from build123d import *

# Parameters (mm, degrees)
SKETCH1_W           = 38
SKETCH1_H           = 38
SKETCH1_R           = 1
BOSS_EXTRUDE1_DEPTH = 2
SKETCH2_R           = 10
BOSS_EXTRUDE2_DEPTH = 5
SKETCH3_R           = 7
BOSS_EXTRUDE3_DEPTH = 17


with BuildPart() as part:
    # Sketch1 → Boss-Extrude1 (new body)
    with BuildSketch(Plane(origin=(0, 0, 0), x_dir=(1, 0, 0), z_dir=(0, 1, 0))):
        Rectangle(SKETCH1_W, SKETCH1_H)
        with Locations(Location((-17, 17, 0), (0, 0, 270))):
            Circle(SKETCH1_R, mode=Mode.SUBTRACT)
        with Locations(Location((17, 17, 0), (0, 0, 270))):
            Circle(SKETCH1_R, mode=Mode.SUBTRACT)
        with Locations(Location((17, -17, 0), (0, 0, 270))):
            Circle(SKETCH1_R, mode=Mode.SUBTRACT)
        with Locations(Location((-17, -17, 0), (0, 0, 270))):
            Circle(SKETCH1_R, mode=Mode.SUBTRACT)
    extrude(amount=BOSS_EXTRUDE1_DEPTH)

    # Sketch2 → Boss-Extrude2 (add)
    with BuildSketch(Plane(origin=(0, 2, 0), x_dir=(1, 0, 0), z_dir=(0, 1, 0))):
        with Locations(Location((0, 0, 0), (0, 0, 270))):
            Circle(SKETCH2_R)
    extrude(amount=BOSS_EXTRUDE2_DEPTH)

    # Sketch3 → Boss-Extrude3 (add)
    with BuildSketch(Plane(origin=(0, 7, 0), x_dir=(1, 0, 0), z_dir=(0, 1, 0))):
        with Locations(Location((0, 0, 0), (0, 0, 270))):
            Circle(SKETCH3_R)
    extrude(amount=BOSS_EXTRUDE3_DEPTH)


solid = part.part
Read the model definition and answer for the solid it produces. Units are mm, in the model's axes. A direction names the side the tool comes from. Coordinates: 2 decimals unless noted, no trailing zeros. Order: outer loops, then holes, each group sorted by start corner. A loop starts at its lowest first (then second) coordinate and runs counter-clockwise, first axis right, second up. Notation, with made-up numbers: (39.25, 47.25) - (80.25, 47.25) arc R7 ccw to (80.25, 54.25) - close; hole circle Ø8 at (10.25, -11.5). An arc over 180 degrees is marked (long way). Use one line per item in the form item = value.
(1) Straight lines are drawn through the part: L1, parallel to X at y = 0.65, z = -17; L2, parallel to Y at x = -3.5, z = 7.5; L3, parallel to Y at x = 15, z = 5.5. For each, find the intervals that lie inside material, in ascending order.
Computed values:
L1 = -19 to -18, -16 to 16, 18 to 19
L2 = 0 to 7
L3 = 0 to 2
(2) For a pull along X with two mould halves and no side action, classify faces 1 (the face through (-19, 1, 0)), 2 (the face through (16, 1, 17)), 3 (the face through (0, 24, 0)) as pulls with the +X half, pulls with the -X half, needs draft (parallel to the pull), parting line crosses it, or undercut.
Computed values:
face_1 = pulls with the -X half
face_2 = undercut
face_3 = needs draft
(3) Section B-B, the plane z = -17 is taken. Give the vertices of the cut face in (x, y), then the cut area to 3 significant figures.
Computed values:
outline = (-19, 0) - (-18, 0) - (-18, 2) - (-19, 2) - close; (-16, 0) - (16, 0) - (16, 2) - (-16, 2) - close; (18, 0) - (19, 0) - (19, 2) - (18, 2) - close
area = 68.0 mm²
(4) Section A-A, the plane x = -17 is taken. Give the vertices of the cut face in (y, z), then the cut area to 3 significant figures.
Computed values:
outline = (0, -19) - (2, -19) - (2, -18) - (0, -18) - close; (0, -16) - (2, -16) - (2, 16) - (0, 16) - close; (0, 18) - (2, 18) - (2, 19) - (0, 19) - close
area = 68.0 mm²
(5) Section D-D, the plane x = 0 is taken. Give the vertices of the cut face in (y, z).
Computed values:
outline = (0, -19) - (2, -19) - (2, -10) - (7, -10) - (7, -7) - (24, -7) - (24, 7) - (7, 7) - (7, 10) - (2, 10) - (2, 19) - (0, 19) - close
(6) Section C-C, the plane z = 0 is taken. Give the vertices of the cut face in (x, y), then the cut area to 3 significant figures.
Computed values:
outline = (-19, 0) - (19, 0) - (19, 2) - (10, 2) - (10, 7) - (7, 7) - (7, 24) - (-7, 24) - (-7, 7) - (-10, 7) - (-10, 2) - (-19, 2) - close
area = 414 mm²
(7) Which of the six approach directions +Z, -Z, +X, -X, +Y, -Y give full straight-line access (tool end or side, diameter ignored) to faces 4 (the face through (0, 0, 0)), 5 (the face through (-9, 2, -9))?
Computed values:
face_4 = +Z, -Z, +X, -X, -Y
face_5 = +Y
(8) Given pin 1 Ø3 at (x, z) = (17, 17) entering from +Y; pin 2 Ø8 at (y, z) = (12, 4.5) entering from -X; pin 3 Ø5 at (y, z) = (7, -4) entering from +X, each flat-ended and moving along its own axis, determine where each tip first touches the part or whether it passes through.
Computed values:
pin_1 = 2
pin_2 = -6.98
pin_3 = 9.89
